Source: CAD feature listing. Evaluate the final solid. Frame: model axes, mm. Round coordinates to 2 decimals unless told otherwise and drop trailing zeros. Put each result on its own line as item: value. Start each with the question number.
1) Line query: probe 1 along Z at (x, y) = (39, 204); probe 2 along Z at (x, y) = (32, 207); probe 3 along X at (y, z) = (235.5, -22) (3 decimals). Output: solid intervals per line, ascending. Write a range as [from, to].
2) Mould query, pull axis X, two halves, no side actions, for faces 1 (the face through (86.4, 216.96, 0.98)), 2 (the face through (90, 195.708, 6)), 3 (the face through (18.967, 217.542, 16.603)), 4 (the face through (162.63, 217.54, 17)). Classes: +X half, -X half, draft (parallel to the pull), parting line (faces both ways), or undercut.
3) Contact query for flat-ended pins moving along their axis: P1, Ø6, axis at y = 208, z = -5, coming from the +X side; P2, Ø1, axis at y = 220.5, z = -16.5, coming from the -X side; P3, Ø5, axis at y = 223, z = -5.5, coming from the +X side (3 decimals). Output: stop coordinate, or through.
```python
from build123d import *

# Parameters (mm, degrees)
BOSS_EXTRUDE1_DEPTH      = 31.75
BOSS_EXTRUDE1_DEPTH_BACK = 31.75
SKETCH1_W                = 182.099207872
SKETCH1_H                = 43.109258089
SKETCH2_W                = 205.659157106
SKETCH2_H                = 99.146034208
CUT_EXTRUDE1_DEPTH       = 190.806723118
SKETCH3_R                = 4.7625
CUT_EXTRUDE2_DEPTH       = 190.806723118
FILLET1_R                = 1.5875


with BuildPart() as part:
    # Sketch1 → Boss-Extrude1 (new, two sides: drawn at the far end of the back side and taken through both)
    with BuildSketch(Plane.XY.offset(-BOSS_EXTRUDE1_DEPTH_BACK)):
        with Locations((91.049603936, 217.262286974)):
            Rectangle(SKETCH1_W, SKETCH1_H)
    extrude(amount=BOSS_EXTRUDE1_DEPTH + BOSS_EXTRUDE1_DEPTH_BACK)

    # Sketch2 → Cut-Extrude1 (cut, through all)
    with BuildSketch(Plane(origin=(0, 238.816916018, 0), x_dir=(1, 0, 0), z_dir=(0, 1, 0))):
        with Locations((89.350434008, 0.474866742)):
            Rectangle(SKETCH2_W, SKETCH2_H)
        with BuildLine():
            Line((1.204268152, -2.540878953), (37.233910096, -31.064345493))
            ThreePointArc((37.233910096, -31.064345493), (38.161341158, -31.573691126), (39.204641944, -31.75))
            Line((39.204641944, -31.75), (142.894565928, -31.75))
            ThreePointArc((142.894565928, -31.75), (143.937866714, -31.573691126), (144.865297776, -31.064345493))
            Line((144.865297776, -31.064345493), (180.894939721, -2.540878953))
            ThreePointArc((180.894939721, -2.540878953), (181.782327763, -1.43420323), (182.099207872, -0.051533461))
            Line((182.099207872, -0.051533461), (182.099207872, 0.051533461))
            ThreePointArc((182.099207872, 0.051533461), (181.782327763, 1.43420323), (180.894939721, 2.540878953))
            Line((180.894939721, 2.540878953), (144.865297776, 31.064345493))
            ThreePointArc((144.865297776, 31.064345493), (143.937866714, 31.573691126), (142.894565928, 31.75))
            Line((142.894565928, 31.75), (39.204641944, 31.75))
            ThreePointArc((39.204641944, 31.75), (38.161341158, 31.573691126), (37.233910096, 31.064345493))
            Line((37.233910096, 31.064345493), (1.204268152, 2.540878953))
            ThreePointArc((1.204268152, 2.540878953), (0.316880109, 1.43420323), (0, 0.051533461))
            Line((0, 0.051533461), (0, -0.051533461))
            ThreePointArc((0, -0.051533461), (0.316880109, -1.43420323), (1.204268152, -2.540878953))
        make_face(mode=Mode.SUBTRACT)
    extrude(amount=-CUT_EXTRUDE1_DEPTH, mode=Mode.SUBTRACT)

    # Sketch3 → Cut-Extrude2 (cut, through all)
    with BuildSketch(Plane.XZ.offset(-195.707657929)):
        with Locations(Location((91.049603936, -0.051533461, 0), (0, 0, 270))):
            Circle(SKETCH3_R)
    extrude(amount=-CUT_EXTRUDE2_DEPTH, mode=Mode.SUBTRACT)

    # Fillet1
    fillet1_edges = [part.edges().sort_by_distance(p)[0] for p in [
        (91.049603936, 195.707657929, 31.75),
        (91.049603936, 238.816916018, 31.75),
        (91.049603936, 238.816916018, -31.75),
        (91.049603936, 195.707657929, -31.75),
        (182.099207872, 195.707657929, 0),
        (0, 195.707657929, 0),
        (182.099207872, 238.816916018, 0),
        (0, 238.816916018, 0),
        (181.782327763, 195.707657929, -1.43420323),
        (162.880118749, 195.707657929, -16.802612223),
        (143.937866714, 195.707657929, -31.573691126),
        (0.316880109, 195.707657929, -1.43420323),
        (38.161341158, 195.707657929, -31.573691126),
        (19.219089124, 195.707657929, -16.802612223),
        (181.782327763, 195.707657929, 1.43420323),
        (143.937866714, 195.707657929, 31.573691126),
        (162.880118749, 195.707657929, 16.802612223),
        (0.316880109, 195.707657929, 1.43420323),
        (19.219089124, 195.707657929, 16.802612223),
        (38.161341158, 195.707657929, 31.573691126),
        (0.316880109, 238.816916018, -1.43420323),
        (19.219089124, 238.816916018, -16.802612223),
        (38.161341158, 238.816916018, -31.573691126),
        (143.937866714, 238.816916018, -31.573691126),
        (162.880118749, 238.816916018, -16.802612223),
        (181.782327763, 238.816916018, -1.43420323),
        (181.782327763, 238.816916018, 1.43420323),
        (162.880118749, 238.816916018, 16.802612223),
        (143.937866714, 238.816916018, 31.573691126),
        (38.161341158, 238.816916018, 31.573691126),
        (19.219089124, 238.816916018, 16.802612223),
        (0.316880109, 238.816916018, 1.43420323),
    ]]
    fillet(fillet1_edges, radius=FILLET1_R)


solid = part.part
```
Answer sheet:
1. probe 1: [-31.74, 31.74]
1. probe 2: [-26.92, 26.92]
1. probe 3: [25.784, 156.315]
2. face 1: undercut
2. face 2: draft
2. face 3: -X half
2. face 4: +X half
3. P1: x = 181.43
3. P2: x = 18.21
3. P3: x = 180.315
